Part print with two shaded views. Sizes in mm from the minimum x, y, z corner. Give positions to 0.01 mm unless a question says otherwise; leave off trailing zeros. Write each loop counter-clockwise with the first axis right and the second up, starting at its lowest first coordinate (ties: lowest second). Pieces come first, ordered by that corner, then holes. Notation, with made-up numbers: (27, 59.5) - (68, 59.5) arc R16 ccw to (68, 72.5) - close; hole circle Ø3 at (16, 14). An arc over 180 degrees is marked (long way). One line per item, written item: value. Start each with the question number.
(1) Cut at B-B, the plane x = 21. List the corners of the cut face in (y, z), and give its area (3 significant figures).
(2) Drop flat-ended pins along their axis: P1, Ø3.5, axis at x = 43.5, y = 1, coming from the -Z side; P2, Ø2.5, axis at x = 10, y = 10.5, coming from the -Z side; P3, Ø4.5, axis at x = 10, z = 5, coming from the +Y side; P4, Ø4, axis at x = 89.5, y = 12, coming from the -Z side. Give the stop position or say it passes through.
(3) Probe L1, parallel to X at y = 1.2, z = 98.53; L2, parallel to X at y = 4, z = 5; L3, parallel to Z at x = 16, y = 5.25. List the from-to ranges inside material, lowest first.
(4) Cut at D-D, the plane z = 180. List the corners of the cut face in (x, y), and give its area (3 significant figures).
(5) Cut at C-C, the plane y = 14.5. List the corners of the cut face in (x, z).
(6) Mould opens along Z. For the marked faces 1 and 2 say: pulls with the +Z half, pulls with the -Z half, needs draft (parallel to the pull), parting line crosses it, or undercut.
(7) Cut at A-A, the plane z = 5. List the corners of the cut face in (x, y).
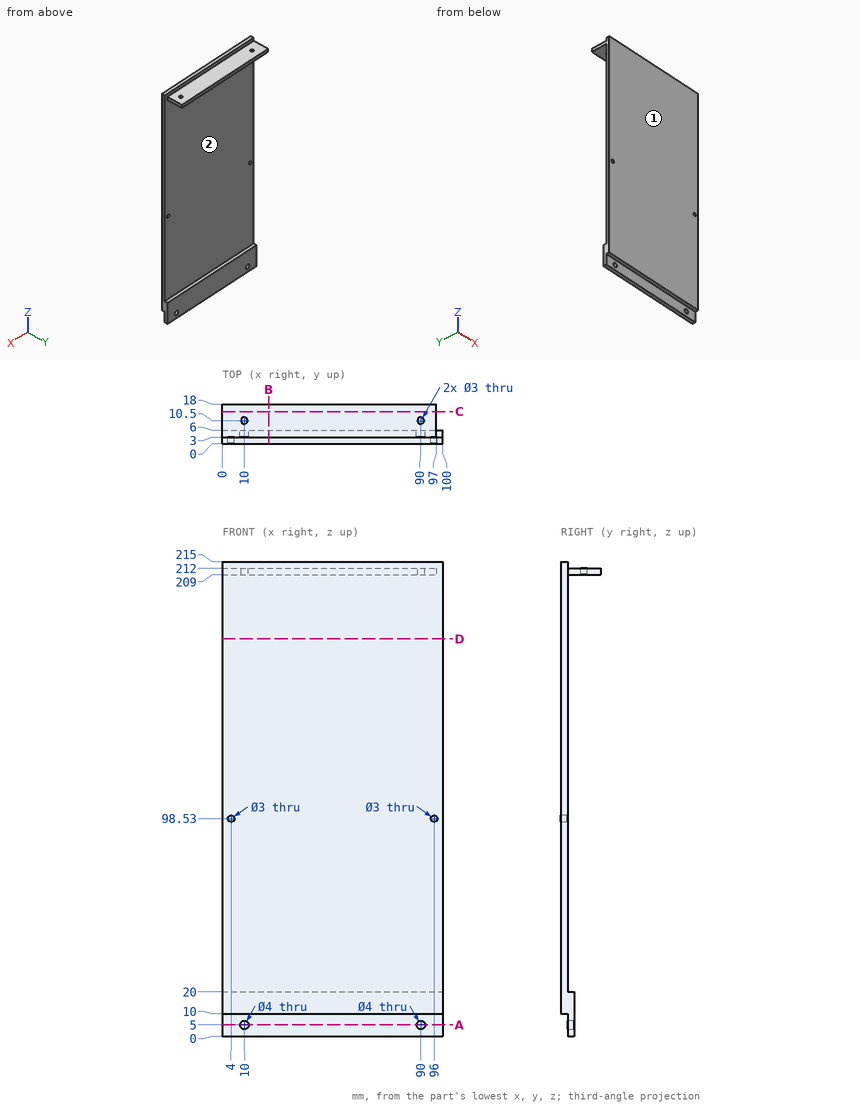
Answers follow:
1. outline: (0, 10) - (3, 10) - (3, 0) - (6, 0) - (6, 20) - (3, 20) - (3, 209) - (18, 209) - (18, 212) - (3, 212) - (3, 215) - (0, 215) - close
1. area: 720 mm²
2. P1: stops at z = 10
2. P2: passes through
2. P3: stops at y = 6
2. P4: stops at z = 209
3. L1: x = 0 to 2.5, 5.5 to 94.5, 97.5 to 100
3. L2: x = 0 to 8, 12 to 88, 92 to 100
3. L3: z = 0 to 20, 209 to 212
4. outline: (0, 0) - (100, 0) - (100, 3) - (0, 3) - close
4. area: 300 mm²
5. outline: (0, 209) - (97, 209) - (97, 212) - (0, 212) - close
6. face 1: needs draft
6. face 2: undercut
7. outline: (0, 3) - (8, 3) - (8, 6) - (0, 6) - close; (12, 3) - (88, 3) - (88, 6) - (12, 6) - close; (92, 3) - (100, 3) - (100, 6) - (92, 6) - close
